Verification items for this drawing (mm, ordinates from the low corner). A direction names the side the tool comes from. Round coordinates to 2 decimals unless told otherwise and drop trailing zeros. Order: outer loops, then holes, each group sorted by start corner. A loop starts at its lowest first (then second) coordinate and runs counter-clockwise, first axis right, second up. Notation, with made-up numbers: M 6,31.5 L 20,31.5 A26 cw 20,53.5 Z; hole C -32,65.25 d8. An arc over 180 degrees is marked long. Use CSV: the item, a comma, the result in double quotes. Start each with the question number.
Q1. Sectioned sample at D-D (z = 58). Enter the section's corners in (x, y), and give its area (3 significant figures).
Q2. Set-up check for the marked faces 1 and 2: record each of +Z, -Z, +X, -X, +Y, -Y from which the full face is reachable in a straight line by a thin tool's end or side.
Q3. Sectioned sample at C-C (z = 32.5). Enter the section's corners in (x, y), and give its area (3 significant figures).
Q4. Sectioned sample at A-A (y = 20). Enter the section's corners in (x, z), and give its area (3 significant figures).
Q5. Scan lines: line 1 (Z direction, x = 1.6, y = 20); line 2 (Z direction, x = 5.5, y = 22); line 3 (X direction, y = 29, z = 49). Record each from-to range of solid material in increasing order.
Q6. Gauge pin test, flat ends, axial feed: pin 1 Ø6 at (y, z) = (15.5, 39.5) entering from +X; pin 2 Ø17.5 at (x, z) = (22, 34) entering from +Y; pin 3 Ø8 at (x, z) = (13.5, 53.5) entering from +Y. Record the tip position at first contact, or that the pin passes through.
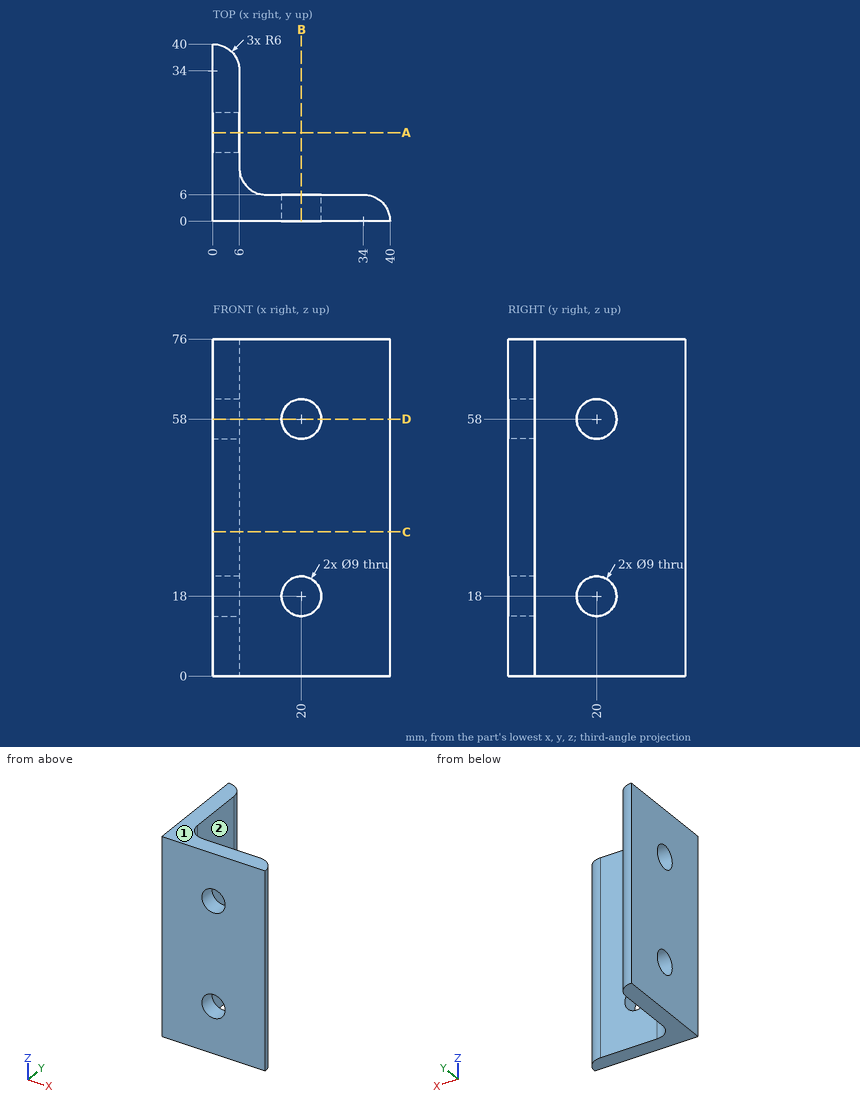
Verdict:
1,outline,"M 0,0 L 15.5,0 L 15.5,6 L 12,6 A6 cw 6,12 L 6,15.5 L 0,15.5 Z; M 0,24.5 L 6,24.5 L 6,34 A6 ccw 0,40 Z; M 24.5,0 L 40,0 A6 ccw 34,6 L 24.5,6 Z"
1,area,"328 mm²"
2,face 1,"+Z, +X, -X, +Y, -Y"
2,face 2,"+Z, -Z, +X, +Y"
3,outline,"M 0,0 L 40,0 A6 ccw 34,6 L 12,6 A6 cw 6,12 L 6,34 A6 ccw 0,40 Z"
3,area,"436 mm²"
4,outline,"M 0,0 L 6,0 L 6,13.5 L 0,13.5 Z; M 0,22.5 L 6,22.5 L 6,53.5 L 0,53.5 Z; M 0,62.5 L 6,62.5 L 6,76 L 0,76 Z"
4,area,"348 mm²"
5,line 1,"z = 0 to 13.5, 22.5 to 53.5, 62.5 to 76"
5,line 2,"z = 0 to 13.97, 22.03 to 53.97, 62.03 to 76"
5,line 3,"x = 0 to 6"
6,pin 1,"stops at x = 6"
6,pin 2,"stops at y = 6"
6,pin 3,"stops at y = 6.55"
